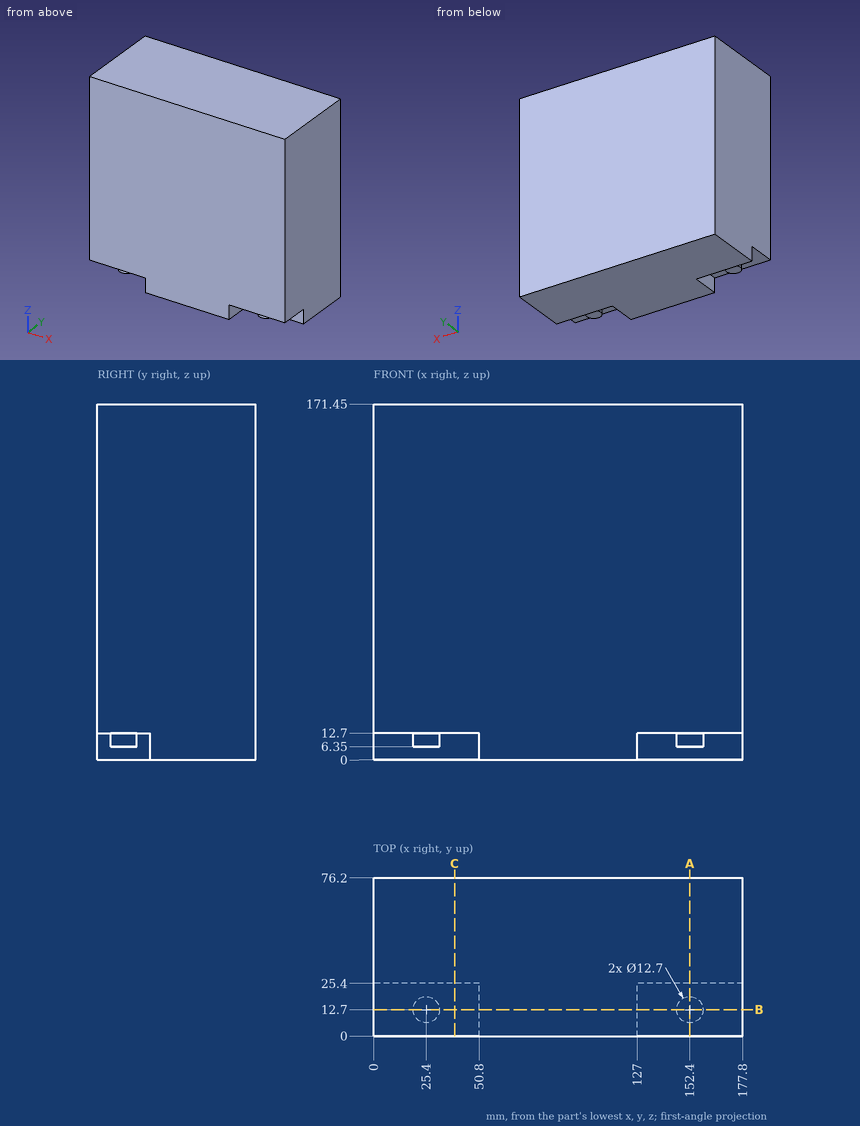
Study the drawing (mm; zero at the part's minimum x, y, z) and answer. Coordinates: 2 decimals unless noted, no trailing zeros. Write each loop counter-clockwise with the first axis right and the second up, starting at its lowest first coordinate (ties: lowest second). Pieces come first, ordered by that corner, then holes. Notation, with made-up numbers: (-3.75, 18) - (50.25, 18) arc R18 ccw to (50.25, 39) - close; hole circle Ø6 at (-40, 48). An arc over 180 degrees is marked (long way). Return JSON: item names as keys, results as strings. Group by question number.
1. A straight line is drawn through the part: L1, parallel to Z at x = 145, y = 11. Find the intervals that lie inside material, in ascending order.
2. A cutting plane is placed at B-B, the plane y = 12.7. Determine the outline of the cut face in (x, z).
3. A cutting plane is placed at A-A, the plane x = 152.4. Determine the outline of the cut face in (y, z).
4. A cutting plane is placed at C-C, the plane x = 39. Determine the outline of the cut face in (y, z).
5. Given pin 1 (4 mm diameter, centred on y = 15, z = 9, fed in from -X); pin 2 (4 mm diameter, centred on y = 13.5, z = 5, fed in from +X); pin 3 (6.5 mm diameter, centred on x = 154, y = 14.5, fed in from -Z); pin 4 (4 mm diameter, centred on x = 97.5, y = 45, fed in from -Z), each flat-ended and moving along its own axis, determine where each tip first touches the part or whether it passes through.
Ans:
{
 "1": {"L1": "12.7 to 171.45"},
 "2": {"outline": "(0, 12.7) - (19.05, 12.7) - (19.05, 6.35) - (31.75, 6.35) - (31.75, 12.7) - (50.8, 12.7) - (50.8, 0) - (127, 0) - (127, 12.7) - (146.05, 12.7) - (146.05, 6.35) - (158.75, 6.35) - (158.75, 12.7) - (177.8, 12.7) - (177.8, 171.45) - (0, 171.45) - close"},
 "3": {"outline": "(0, 12.7) - (6.35, 12.7) - (6.35, 6.35) - (19.05, 6.35) - (19.05, 12.7) - (25.4, 12.7) - (25.4, 0) - (76.2, 0) - (76.2, 171.45) - (0, 171.45) - close"},
 "4": {"outline": "(0, 12.7) - (25.4, 12.7) - (25.4, 0) - (76.2, 0) - (76.2, 171.45) - (0, 171.45) - close"},
 "5": {"pin 1": "x = 19.06", "pin 2": "x = 158.75", "pin 3": "z = 6.35", "pin 4": "z = 0"}
}
